Read the model definition and answer for the solid it produces. Units are mm, in the model's axes. A direction names the side the tool comes from. Give positions to 0.01 mm unless a question says otherwise; leave off trailing zeros. Write each loop counter-clockwise with the first axis right and the second up, starting at its lowest first coordinate (ties: lowest second). Pieces come first, ordered by that corner, then holes. Notation, with made-up numbers: M 54,88 L 97,88 A21 ccw 97,111 Z; hole C 78.25,-33.75 d4. An arc over 180 degrees is marked long. Use a Markdown table: item, result. Add a question column.
Item 1: A cutting plane is placed at D-D on x = -1.75. Determine the outline of the cut face in (y, z), then the cut area to 3 significant figures.
Item 2: A cutting plane is placed at B-B on z = -10. Determine the outline of the cut face in (x, y).
Item 3: A cutting plane is placed at A-A on x = -8. Determine the outline of the cut face in (y, z), then the cut area to 3 significant figures.
Item 4: Consider probe 1 along Z at (x, y) = (8, 1.1). Determine where the line is inside the solid, lowest interval first. Write a range as [from, to].
Item 5: Given P1, Ø5, axis at x = 4.5, z = -1, coming from the -Y side; P2, Ø0.9, axis at x = 6, y = 0.5, coming from the -Z side; P3, Ø0.5, axis at x = 5.5, y = 1, coming from the +Z side; P4, Ø0.5, axis at y = 1, z = 7, coming from the +X side, each flat-ended and moving along its own axis, determine where each tip first touches the part or whether it passes through.
Item 6: For faces 5 (the flat face through (7, 1, -2.75)), 6 (the flat face through (-2.75, 1, -7)), 7 (the flat face through (-2.75, 1, 7)), 8 (the cylindrical face through (-5.61, 0.86, -0.12)), determine the directions among +Z, -Z, +X, -X, +Y, -Y from which every point of the face is accessible in a straight line to the end or side of a thin tool.
Item 7: A cutting plane is placed at C-C on y = 2.15. Determine the outline of the cut face in (x, z).
Item 8: The mould has two halves that part along X. Classify faces 1 (the cylindrical face through (-1.998, 0.887, 13.787)), 2 (the cylindrical face through (0.018, 0.863, -12.406)), 3 (the cylindrical face through (-0.018, 0.863, 10.406)), 4 (the flat face through (2.75, 1, 7)): pulls with the +X half, pulls with the -X half, needs draft (parallel to the pull), parting line crosses it, or undercut.
from build123d import *

# Parameters (mm, degrees)
SKETCH1_W                = 5.5
SKETCH1_H                = 14.5
SKETCH1_R                = 0.4064
BOSS_EXTRUDE1_DEPTH      = 1.75
FILLET1_R                = 2.5
CIRPATTERN1_COUNT        = 4
FILLET1_OF_CIRPATTERN1_R = 2.5
CUT_EXTRUDE1_REACH       = 22.581
SKETCH2_R                = 1
BOSS_EXTRUDE2_START      = 1.25
SKETCH3_R                = 3
SKETCH3_R_2              = 1
BOSS_EXTRUDE2_DEPTH      = 1.25


with BuildPart() as part:
    # Sketch1 → Boss-Extrude1 (new body)
    with BuildSketch(Plane(origin=(0, 0, 0), x_dir=(1, 0, 0), z_dir=(0, 1, 0))):
        with Locations((0, 7.25)):
            Rectangle(SKETCH1_W, SKETCH1_H)
        with Locations(Location((0, 12, 0), (0, 0, 270))):
            Circle(SKETCH1_R, mode=Mode.SUBTRACT)
        with Locations(Location((0, 10, 0), (0, 0, 270))):
            Circle(SKETCH1_R, mode=Mode.SUBTRACT)
        with Locations(Location((0, 8, 0), (0, 0, 270))):
            Circle(SKETCH1_R, mode=Mode.SUBTRACT)
        with Locations(Location((0, 6, 0), (0, 0, 270))):
            Circle(SKETCH1_R, mode=Mode.SUBTRACT)
    boss_extrude1 = extrude(amount=BOSS_EXTRUDE1_DEPTH)

    # Fillet1
    fillet1_edges = [part.edges().sort_by_distance(p)[0] for p in [
        (-2.75, 0.875, -14.5),
        (2.75, 0.875, -14.5),
    ]]
    fillet(fillet1_edges, radius=FILLET1_R)

    # CirPattern1: Boss-Extrude1 ×4 about axis
    cirpattern1_axis = Axis((0, 0, 0), (0, 1, 0))
    for i in range(1, CIRPATTERN1_COUNT):
        add(boss_extrude1.rotate(cirpattern1_axis, i * 360 / CIRPATTERN1_COUNT))

    # Fillet1 of CirPattern1
    fillet1_of_cirpattern1_edges = [part.edges().sort_by_distance(p)[0] for p in [
        (-14.5, 0.875, 2.75),
        (-14.5, 0.875, -2.75),
        (2.75, 0.875, 14.5),
        (-2.75, 0.875, 14.5),
        (14.5, 0.875, -2.75),
        (14.5, 0.875, 2.75),
    ]]
    fillet(fillet1_of_cirpattern1_edges, radius=FILLET1_OF_CIRPATTERN1_R)

    # Sketch2 → Cut-Extrude1 (cut, up to next)
    with BuildSketch(Plane(origin=(0, 1.75, 0), x_dir=(1, 0, 0), z_dir=(0, 1, 0)), mode=Mode.PRIVATE) as cut_extrude1_sk1:
        with Locations(Location((0, 0, 0), (0, 0, 270))):
            Circle(SKETCH2_R)
    cut_extrude1_tool1 = extrude(cut_extrude1_sk1.sketch, amount=-CUT_EXTRUDE1_REACH, mode=Mode.PRIVATE) & part.part
    add(cut_extrude1_tool1.solids().sort_by_distance((0, 1.75, 0))[0], mode=Mode.SUBTRACT)

    # Sketch3 → Boss-Extrude2 (add)
    with BuildSketch(Plane(origin=(0, 1.75, 0), x_dir=(1, 0, 0), z_dir=(0, 1, 0)).offset(BOSS_EXTRUDE2_START)):
        with Locations(Location((0, 0, 0), (0, 0, 270))):
            Circle(SKETCH3_R)
        with Locations(Location((0, 0, 0), (0, 0, 270))):
            Circle(SKETCH3_R_2, mode=Mode.SUBTRACT)
    extrude(amount=-BOSS_EXTRUDE2_DEPTH)


solid = part.part
Filled in:
| question | item | result |
|---|---|---|
| 1 | outline | M 0,-14 L 1.75,-14 L 1.75,-2.44 L 3,-2.44 L 3,2.44 L 1.75,2.44 L 1.75,14 L 0,14 Z |
| 1 | area | 55.1 mm² |
| 2 | outline | M -2.75,0 L -0.41,0 L -0.41,1.75 L -2.75,1.75 Z; M 0.41,0 L 2.75,0 L 2.75,1.75 L 0.41,1.75 Z |
| 3 | outline | M 0,-2.75 L 1.75,-2.75 L 1.75,-0.41 L 0,-0.41 Z; M 0,0.41 L 1.75,0.41 L 1.75,2.75 L 0,2.75 Z |
| 3 | area | 8.20 mm² |
| 4 | probe 1 | [-2.75, -0.41], [0.41, 2.75] |
| 5 | P1 | y = 0 |
| 5 | P2 | z = -2.75 |
| 5 | P3 | z = 2.75 |
| 5 | P4 | x = 2.75 |
| 6 | face 5 | -Z, +X, +Y, -Y |
| 6 | face 6 | -Z, -X, +Y, -Y |
| 6 | face 7 | +Z, -X, +Y, -Y |
| 6 | face 8 | +Y, -Y |
| 7 | outline | C 0,0 d6; hole C 0,0 d2 |
| 8 | face 1 | pulls with the -X half |
| 8 | face 2 | undercut |
| 8 | face 3 | undercut |
| 8 | face 4 | pulls with the +X half |
